Design review of the part built by this model. Coordinates are the model's own, in mm. A direction names the side the tool comes from. Give positions to 0.01 mm unless a question says otherwise; leave off trailing zeros. Order: outer loops, then holes, each group sorted by start corner. A loop starts at its lowest first (then second) coordinate and runs counter-clockwise, first axis right, second up. Notation, with made-up numbers: (86.25, 8) -> (113.25, 8) arc R20 ccw to (113.25, 46) -> close; hole circle Ø8 at (88.25, 3). An arc over 180 degrees is marked (long way). One line per item, written item: value. Start each with the question number.
1) Consider section C-C (y = -8). State the section outline as (x, z) points.
2) Consider section D-D (y = 23). State the section outline as (x, z) points.
3) The part is to be moulded in two halves that separate along Z. For faces 3 (the face through (60.996, -15.789, 33.061)), 4 (the face through (0, -7, 18)), 5 (the face through (31, 8, 31.348)), say which applies: released by +Z, released by -Z, zero draft, split by the parting line, or undercut.
4) For pin 1 (8 mm diameter, centred on x = 20, y = -10, fed in from +Z); pin 2 (1.5 mm diameter, centred on x = 49.5, z = 43, fed in from -Y); pin 3 (1.5 mm diameter, centred on x = 54, y = -10.5, fed in from +Z), all flat-tipped, find the tip position at first contact; note any pin that passes through.
5) Tool access review of faces 1 (the face through (31.306, 11.913, 30.142)), 2 (the face through (61.56, -27.97, 4.71)): name each direction out of +Z, -Z, +X, -X, +Y, -Y from which nothing blocks a thin tool from reaching the whole face with its end or side.
6) Consider section A-A (x = 51). State the section outline as (y, z) points, plus the area to 3 significant figures.
7) Wall thickness on line 1 along Y through (x, z) = (27.5, 10.5); line 2 along Z through (x, y) = (17.5, 3.5); line 3 along Y through (x, z) = (22.5, 34): over which ranges is each line inside the solid? List them lowest first. Write a range as from..to.
8) Consider section B-B (z = 24). State the section outline as (x, y) points.
from build123d import *

# Parameters (mm, degrees)
F1_DEPTH = 63.5
F2_SIZE  = 5.08


with BuildPart() as f1:
    # F0 (on Right) → F1 (new body)
    with BuildSketch(Plane.YZ):
        with BuildLine():
            ThreePointArc((-30.862735, 9.241248), (-30.625866, 3.03616), (-25.209136, 0))
            Line((-25.209136, 0), (25.209136, 0))
            ThreePointArc((25.209136, 0), (30.625866, 3.03616), (30.862735, 9.241248))
            Line((30.862735, 9.241248), (5.653599, 58.535651))
            ThreePointArc((5.653599, 58.535651), (0, 61.994403), (-5.653599, 58.535651))
            Line((-5.653599, 58.535651), (-30.862735, 9.241248))
        make_face()
        with BuildLine():
            ThreePointArc((2.236106, 9.505495), (0, 8.170248), (-2.236106, 9.505495))
            Line((-2.236106, 9.505495), (-11.986921, 27.603697))
            ThreePointArc((-11.986921, 27.603697), (-11.931603, 30.110665), (-9.750815, 31.348449))
            Line((-9.750815, 31.348449), (-6.28835, 31.348449))
            ThreePointArc((-6.28835, 31.348449), (-4.492299, 32.092398), (-3.74835, 33.888449))
            Line((-3.74835, 33.888449), (-3.74835, 49.257109))
            ThreePointArc((-3.74835, 49.257109), (-3.004401, 51.05316), (-1.20835, 51.797109))
            Line((-1.20835, 51.797109), (1.20835, 51.797109))
            ThreePointArc((1.20835, 51.797109), (3.004401, 51.05316), (3.74835, 49.257109))
            Line((3.74835, 49.257109), (3.74835, 33.888449))
            ThreePointArc((3.74835, 33.888449), (4.492299, 32.092398), (6.28835, 31.348449))
            Line((6.28835, 31.348449), (9.750815, 31.348449))
            ThreePointArc((9.750815, 31.348449), (11.931603, 30.110665), (11.986921, 27.603697))
            Line((11.986921, 27.603697), (2.236106, 9.505495))
        make_face(mode=Mode.SUBTRACT)
    extrude(amount=F1_DEPTH)

    # F2
    f2_edges = [f1.edges().sort_by_distance(p)[0] for p in [
        (63.5, 0, 0),
    ]]
    chamfer(f2_edges, length=F2_SIZE)


solid = f1.part
Checked values:
1. outline: (0, 0) -> (58.42, 0) -> (63.5, 5.08) -> (63.5, 20.2) -> (0, 20.2) -> close; (0, 31.35) -> (63.5, 31.35) -> (63.5, 42.79) -> (58.42, 53.95) -> (0, 53.95) -> close
2. outline: (0, 0) -> (58.42, 0) -> (63.5, 5.08) -> (63.5, 13.46) -> (58.42, 24.62) -> (0, 24.62) -> close
3. face 3: released by +Z
3. face 4: zero draft
3. face 5: undercut
4. pin 1: stops at z = 57.86
4. pin 2: stops at y = -13.98
4. pin 3: stops at z = 50.53
5. face 1: +X, -X
5. face 2: +X, -Y
6. outline: (-30.86, 9.24) arc R6.35 ccw to (-25.21, 0) -> (25.21, 0) arc R6.35 ccw to (30.86, 9.24) -> (5.65, 58.54) arc R6.35 ccw to (-5.65, 58.54) -> close; hole (-11.99, 27.6) -> (-2.24, 9.51) arc R2.54 ccw to (2.24, 9.51) -> (11.99, 27.6) arc R2.54 ccw to (9.75, 31.35) -> (6.29, 31.35) arc R2.54 cw to (3.75, 33.89) -> (3.75, 49.26) arc R2.54 ccw to (1.21, 51.8) -> (-1.21, 51.8) arc R2.54 ccw to (-3.75, 49.26) -> (-3.75, 33.89) arc R2.54 cw to (-6.29, 31.35) -> (-9.75, 31.35) arc R2.54 ccw to start
6. area: 1,890 mm^2
7. line 1: y = -30.22..-2.77, 2.77..30.22
7. line 2: z = 0..11.85, 50.35..60.94
7. line 3: y = -18.2..-3.75, 3.75..18.2
8. outline: (0, -23.32) -> (58.42, -23.32) -> (63.5, -17.61) -> (63.5, -10.05) -> (0, -10.05) -> close; (0, 10.05) -> (63.5, 10.05) -> (63.5, 17.61) -> (58.42, 23.32) -> (0, 23.32) -> close
